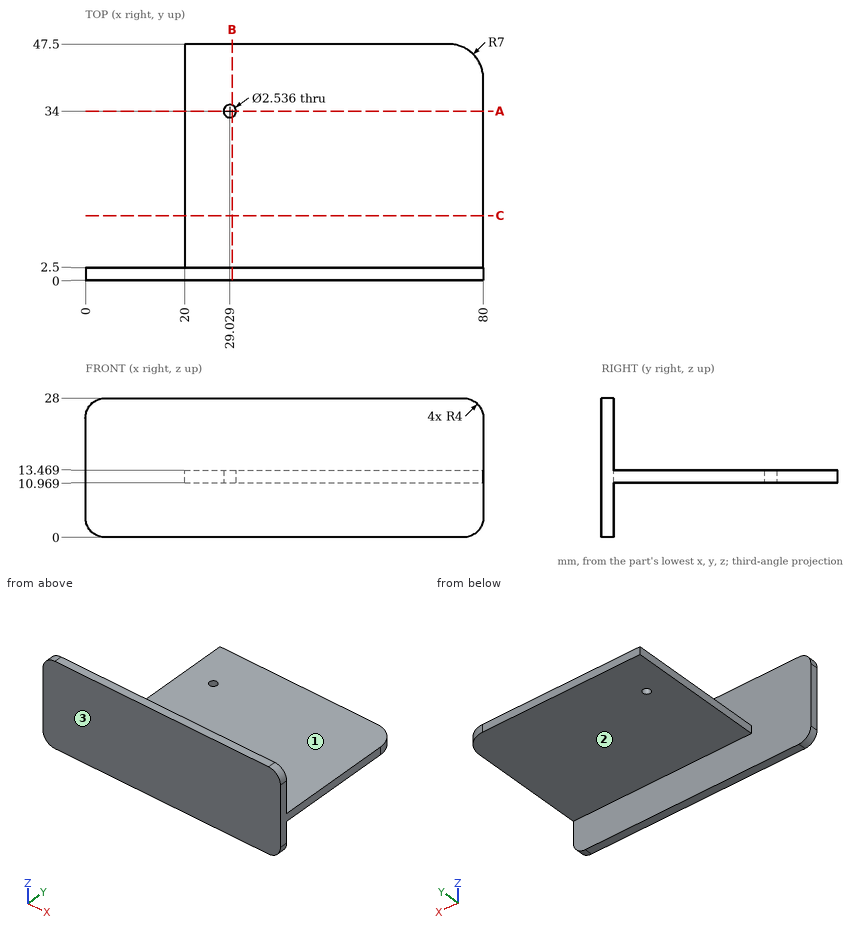
Verification items for this drawing (mm, ordinates from the low corner). A direction names the side the tool comes from. Give positions to 0.01 mm unless a question says otherwise; leave off trailing zeros. Loops run counter-clockwise (first coordinate to the right, second up) from the corner with the lowest first, then second, coordinate; pieces in that order, holes last. Notation, with made-up numbers: (23.5, -32.5) - (59.5, -32.5) arc R36 cw to (59.5, 1.5) - close; hole circle Ø3 at (-39.5, 45.25). An arc over 180 degrees is marked (long way). Write item = value, one per line. Start each with the question number.
Q1. Cross-section at A-A, the plane y = 34. Enter the section's corners in (x, z), and give its area (3 significant figures).
Q2. Depth check by flat-ended pin: P1, Ø4, axis at x = 29.03, y = 34, coming from the +Z side; P2, Ø6, axis at y = 16.5, z = 18, coming from the +X side; P3, Ø10, axis at y = 18.5, z = 12, coming from the -X side; P4, Ø5, axis at x = 35.5, y = 13, coming from the -Z side. Enter the tip coordinate at first touch or a pass-through.
Q3. Cross-section at C-C, the plane y = 13. Enter the section's corners in (x, z), and give its area (3 significant figures).
Q4. Thickness scan on line 1 (X direction, y = 34, z = 12); line 2 (Y direction, x = 9, z = 13.75); line 3 (Z direction, x = 72.5, y = 36.5). Record the ranges inside material, lowest first.
Q5. Tool access check on the marked faces 1, 2 and 3. Record the directions out of +Z, -Z, +X, -X, +Y, -Y that give a thin tool (end or side, any length) a straight path to the whole face; none if there is none.
Q6. Cross-section at B-B, the plane x = 29.5. Enter the section's corners in (y, z).
Answer key:
q1.outline = (20, 10.97) - (27.76, 10.97) - (27.76, 13.47) - (20, 13.47) - close; (30.3, 10.97) - (80, 10.97) - (80, 13.47) - (30.3, 13.47) - close
q1.area = 144 mm^2
q2.P1 = 13.47
q2.P2 = through
q2.P3 = 20
q2.P4 = 10.97
q3.outline = (20, 10.97) - (80, 10.97) - (80, 13.47) - (20, 13.47) - close
q3.area = 150 mm^2
q4.line_1 = 20 to 27.76, 30.3 to 80
q4.line_2 = 0 to 2.5
q4.line_3 = 10.97 to 13.47
q5.face_1 = +Z, +X, -X, +Y
q5.face_2 = -Z, +X, -X, +Y
q5.face_3 = +Z, -Z, +X, -X, -Y
q6.outline = (0, 0) - (2.5, 0) - (2.5, 10.97) - (32.82, 10.97) - (32.82, 13.47) - (2.5, 13.47) - (2.5, 28) - (0, 28) - close; (35.18, 10.97) - (47.5, 10.97) - (47.5, 13.47) - (35.18, 13.47) - close
